```python
from build123d import *

# Parameters (mm, degrees)
SKETCH1_R           = 2
BOSS_EXTRUDE1_DEPTH = 3.175


with BuildPart() as part:
    # Sketch1 → Boss-Extrude1 (new, symmetric)
    with BuildSketch(Plane(origin=(0, 0, 0), x_dir=(1, 0, 0), z_dir=(0, 1, 0))):
        Polygon((-81.35, -18.175), (81.35, -18.175), (81.35, 1.825), (75, 1.825), (75, 11.825), (10, 11.825), (10, 18.175), (-10, 18.175), (-10, 11.825), (-75, 11.825), (-75, 1.825), (-81.35, 1.825), align=None)
        with Locations(Location((-50, -8.175, 0), (0, 0, 270))):
            Circle(SKETCH1_R, mode=Mode.SUBTRACT)
        with Locations(Location((50, -8.175, 0), (0, 0, 270))):
            Circle(SKETCH1_R, mode=Mode.SUBTRACT)
    extrude(amount=BOSS_EXTRUDE1_DEPTH, both=True)


solid = part.part
```
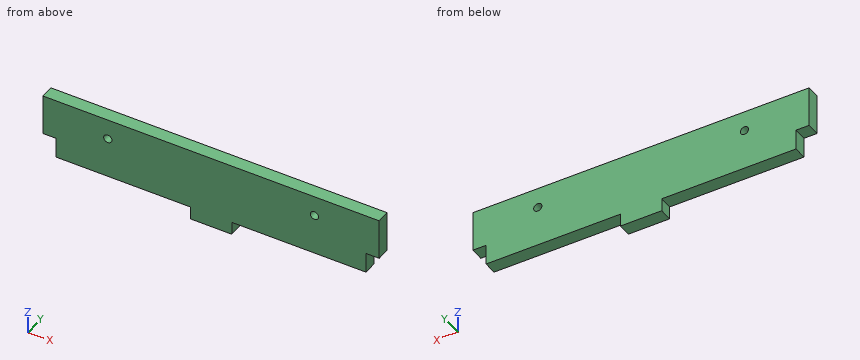
Geometry: final body of the model. Coordinates: model frame, mm. Round coordinates to 2 decimals unless told otherwise and drop trailing zeros. Order: outer loops, then holes, each group sorted by start corner. A loop starts at its lowest first (then second) coordinate and runs counter-clockwise, first axis right, second up. Notation, with made-up numbers: (21, 23.5) - (59, 23.5) arc R26 ccw to (59, 58.5) - close; hole circle Ø5 at (71, 4.25). An arc over 180 degrees is marked (long way). Use CSV: the item, a comma, the result in double quotes. Start each with the question number.
Q1. Section query B-B (y = 2). Return loops of the section in (x, z) (3 decimals).
Q2. Section query C-C (x = -11.5). Return loops of the section in (y, z) (3 decimals), and give its area (4 significant figures).
Q3. Section query D-D (z = -4). Return loops of the section in (x, y) (3 decimals), and give its area (4 significant figures).
Q4. First-contact query: pin 1 (1.9 mm diameter, centred on x = 52, y = 0, fed in from -Z) (3 decimals); pin 2 (6.5 mm diameter, centred on x = 50, z = 8.175, fed in from +Y) (3 decimals); pin 3 (3 mm diameter, centred on y = 0, z = -9, fed in from -X); pin 4 (3 mm diameter, centred on x = 79, y = 1, fed in from -Z) (3 decimals). Flat tips, straight axial feed; report the tip coordinate or a pass-through.
Q5. Section query A-A (x = -50). Return loops of the section in (y, z) (3 decimals), and give its area (3 significant figures).
Q6. Material intervals for line 1 along X through (y, z) = (2.25, 7); line 2 along X through (y, z) = (-1, -13.5); line 3 along X through (y, z) = (2, -5.5), sorted ascending. Write a range as from..to.
Result set:
1,outline,"(-81.35, -1.825) - (-75, -1.825) - (-75, -11.825) - (-10, -11.825) - (-10, -18.175) - (10, -18.175) - (10, -11.825) - (75, -11.825) - (75, -1.825) - (81.35, -1.825) - (81.35, 18.175) - (-81.35, 18.175) - close; hole circle Ø4 at (-50, 8.175); hole circle Ø4 at (50, 8.175)"
2,outline,"(-3.175, -11.825) - (3.175, -11.825) - (3.175, 18.175) - (-3.175, 18.175) - close"
2,area,"190.5 mm2"
3,outline,"(-75, -3.175) - (75, -3.175) - (75, 3.175) - (-75, 3.175) - close"
3,area,"952.5 mm2"
4,pin 1,"stops at z = -11.825"
4,pin 2,"stops at y = 3.175"
4,pin 3,"stops at x = -75"
4,pin 4,"stops at z = -1.825"
5,outline,"(-3.175, -11.825) - (3.175, -11.825) - (3.175, 6.175) - (-3.175, 6.175) - close; (-3.175, 10.175) - (3.175, 10.175) - (3.175, 18.175) - (-3.175, 18.175) - close"
5,area,"165 mm2"
6,line 1,"x = -81.35..-51.62, -48.38..48.38, 51.62..81.35"
6,line 2,"x = -10..10"
6,line 3,"x = -75..75"
